```python
from build123d import *

# Parameters (mm, degrees)
SKETCH2_R           = 9
BOSS_EXTRUDE1_DEPTH = 3
SKETCH3_R           = 6
CUT_EXTRUDE1_DEPTH  = 6
SKETCH4_R           = 8.5
SKETCH4_R_2         = 7.5
SKETCH4_R_3         = 6.5
CUT_EXTRUDE2_DEPTH  = 0.5


with BuildPart() as part:
    # Sketch2 → Boss-Extrude1 (new, symmetric)
    with BuildSketch(Plane(origin=(0, 0, 0), x_dir=(0, 0, -1), z_dir=(1, 0, 0))):
        Circle(SKETCH2_R)
    extrude(amount=BOSS_EXTRUDE1_DEPTH, both=True)

    # Sketch3 → Cut-Extrude1 (cut)
    with BuildSketch(Plane(origin=(3, 0, 0), x_dir=(0, 0, -1), z_dir=(1, 0, 0))):
        Circle(SKETCH3_R)
    extrude(amount=-CUT_EXTRUDE1_DEPTH, mode=Mode.SUBTRACT)

    # Sketch4 → Cut-Extrude2 (cut)
    with BuildSketch(Plane(origin=(3, 0, 0), x_dir=(0, 0, -1), z_dir=(1, 0, 0))):
        Circle(SKETCH4_R)
        Circle(SKETCH4_R_2, mode=Mode.SUBTRACT)
        Circle(SKETCH4_R_2)
        Circle(SKETCH4_R_3, mode=Mode.SUBTRACT)
    cut_extrude2 = extrude(amount=-CUT_EXTRUDE2_DEPTH, mode=Mode.SUBTRACT)

    # Mirror1: Cut-Extrude2 across plane
    add(cut_extrude2.mirror(Plane(origin=(0, 0, 0), x_dir=(0, 0, 1), z_dir=(1, 0, 0))), mode=Mode.SUBTRACT)


solid = part.part
```
Can you work these out from the model? Positions are in its coordinate system, mm. A direction names the side the tool comes from. Give positions to 0.01 mm unless a question says otherwise; leave off trailing zeros. Loops run counter-clockwise (first coordinate to the right, second up) from the corner with the lowest first, then second, coordinate; pieces in that order, holes last. Notation, with made-up numbers: M -34.5,82 L 23.5,82 A25 ccw 23.5,99 Z; hole C 67.25,30.25 d4. An arc over 180 degrees is marked long. Use CSV: the item, a comma, the result in double quotes. Start each with the question number.
1. Imagine slicing it at D-D, the plane z = -7.5. Write out the boundary of the cut face in (x, y), plus the area to 3 significant figures.
2. If we mould it in two halves opening along Z, with no side actions, what happens to faces 1 (the face through (0.042, 8.923, 1.172)), 2 (the face through (2.754, 7.167, -4.57)), 3 (the face through (-3, -3.3, -8))? For each: released by +Z, released by -Z, zero draft, split by the parting line, or undercut.
3. If I drill on L1, parallel to Y at x = 0.95, z = 0; L2, parallel to Y at x = 2.65, z = -4.25; L3, parallel to X at y = -8, z = 2, over which ranges is the centre line in solid material (lowest first)?
4. For P1, Ø1.5, axis at x = -2, z = -5, coming from the +Y side; P2, Ø1, axis at y = -6, z = 4.5, coming from the +X side; P3, Ø1, axis at x = -2, y = -4.5, coming from the +Z side, each with a flat end and sliding along its axis, tell me the tip position at first contact or that it passes through.
5. Imagine slicing it at A-A, the plane y = 0. Write out the boundary of the cut face in (x, z), plus the area to 3 significant figures.
6. On a 3-axis mill with a long thin cutter (end or side, diameter ignored), from which of +Z, -Z, +X, -X, +Y, -Y can I reach the whole of each face in a straight line? I mean faces 4 (the face through (-2.754, 7.167, -4.57)), 5 (the face through (2.754, -3.955, 5.158)), 6 (the face through (-3, -6, -2)). Say none if no direction works.
7. Imagine slicing it at C-C, the plane x = 1. Write out the boundary of the cut face in (y, z).
Response values:
1,outline,"M -3,-4.97 L 3,-4.97 L 3,-4 L 2.5,-4 L 2.5,4 L 3,4 L 3,4.97 L -3,4.97 L -3,4 L -2.5,4 L -2.5,-4 L -3,-4 Z"
1,area,"51.7 mm^2"
2,face 1,"split by the parting line"
2,face 2,"undercut"
2,face 3,"zero draft"
3,L1,"-9 to -6, 6 to 9"
3,L2,"-7.93 to -7.36, -4.92 to -4.24, 4.24 to 4.92, 7.36 to 7.93"
3,L3,"-2.5 to 2.5"
4,P1,"y = 7.93"
4,P2,"x = 2.5"
4,P3,"z = 8.06"
5,outline,"M -3,-9 L 3,-9 L 3,-8.5 L 2.5,-8.5 L 2.5,-6.5 L 3,-6.5 L 3,-6 L -3,-6 L -3,-6.5 L -2.5,-6.5 L -2.5,-8.5 L -3,-8.5 Z; M -3,6 L 3,6 L 3,6.5 L 2.5,6.5 L 2.5,8.5 L 3,8.5 L 3,9 L -3,9 L -3,8.5 L -2.5,8.5 L -2.5,6.5 L -3,6.5 Z"
5,area,"32.0 mm^2"
6,face 4,"-X"
6,face 5,"+X"
6,face 6,"+Z, -Z, -X, +Y, -Y"
7,outline,"C 0,0 d18; hole C 0,0 d12"
